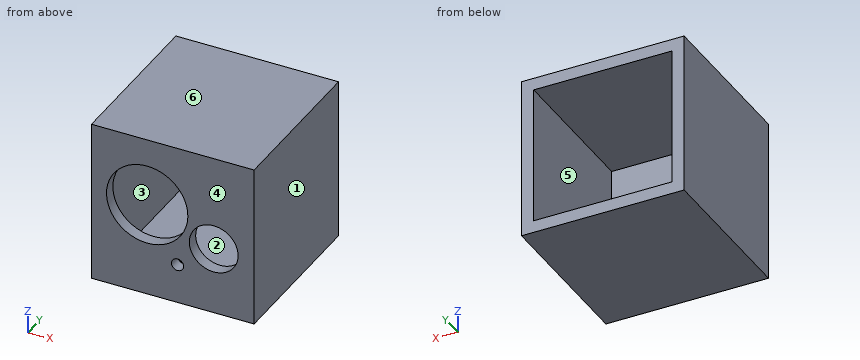
```python
from build123d import *

# Parameters (mm, degrees)
SKETCH1_W           = 20
SKETCH1_H           = 20
BOSS_EXTRUDE1_DEPTH = 20
SHELL1_T            = -1.5
SKETCH2_R           = 5
SKETCH2_R_2         = 0.75
SKETCH2_R_3         = 3
CUT_EXTRUDE1_DEPTH  = 35.641016151


with BuildPart() as part:
    # Sketch1 → Boss-Extrude1 (new body)
    with BuildSketch(Plane(origin=(0, 0, 0), x_dir=(1, 0, 0), z_dir=(0, 1, 0))):
        with Locations((-10, 10)):
            Rectangle(SKETCH1_W, SKETCH1_H)
    extrude(amount=BOSS_EXTRUDE1_DEPTH)

    # Shell1
    shell1_openings = [part.faces().sort_by_distance(p)[0] for p in [
        (-10, 20, -10),
    ]]
    offset(amount=SHELL1_T, openings=shell1_openings, kind=Kind.INTERSECTION)

    # Sketch2 → Cut-Extrude1 (cut, through all)
    with BuildSketch(Plane.XZ):
        with Locations(Location((-13.147042084, -8.401387365, 0), (0, 0, 270))):
            Circle(SKETCH2_R)
        with Locations(Location((-9.417853088, -15.104070699, 0), (0, 0, 270))):
            Circle(SKETCH2_R_2)
        with Locations(Location((-4.966731055, -11.717786539, 0), (0, 0, 270))):
            Circle(SKETCH2_R_3)
    extrude(amount=-CUT_EXTRUDE1_DEPTH, mode=Mode.SUBTRACT)


solid = part.part
```
Source: CAD feature listing. Evaluate the final solid. Frame: model axes, mm. Face numbers are marked on the shaded views. A direction names the side the tool comes from. Coordinates: 2 decimals unless noted, no trailing zeros. Order: outer loops, then holes, each group sorted by start corner. A loop starts at its lowest first (then second) coordinate and runs counter-clockwise, first axis right, second up. Notation, with made-up numbers: M 51,48.25 L 69,48.25 A13 cw 69,73.25 Z; hole C 65,79 d11. An arc over 180 degrees is marked long. Write each question's results on one line, items separated by ' | '. Start each with the question number.
1) Section query D-D (z = -16.5). Return the cut outline in (x, y).
2) Section query B-B (x = -2.75). Return the cut outline in (y, z), plus the area to 3 significant figures.
3) Access query for the marked faces 5 and 6. Directions: +Z, -Z, +X, -X, +Y, -Y. A direction counts if a zero-diameter tool reaches every point of the face in a straight line with its end or side. Return the directions, or none.
4) Section query C-C (z = -5.5). Return the cut outline in (x, y).
5) Line query: line 1 (Z direction, x = -10, y = 16); line 2 (X direction, y = 1, z = -11). Output: solid intervals per line, ascending. Write a range as from..to.
6) Draft query along X for the marked faces 1, 2, 3 and 4. Return one class per face: released by +X, released by -X, zero draft, split by the parting line, or undercut.
7) Section query A-A (y = 6.75). Return the cut outline in (x, z), plus the area to 3 significant figures.
8) Contact query for flat-ended pins moving along their axis: pin 1 Ø5 at (x, y) = (-15.5, 16.5) entering from +Z; pin 2 Ø5 at (x, z) = (-6.5, -11) entering from +Y. Output: stop coordinate, or through.
Answers:
1) outline: M -20,0 L 0,0 L 0,20 L -1.5,20 L -1.5,1.5 L -18.5,1.5 L -18.5,20 L -20,20 Z
2) outline: M 0,-20 L 20,-20 L 20,-18.5 L 1.5,-18.5 L 1.5,-13.74 L 0,-13.74 Z; M 0,-9.7 L 1.5,-9.7 L 1.5,-1.5 L 20,-1.5 L 20,0 L 0,0 Z | area: 79.4 mm^2
3) face 5: +Y | face 6: +Z, +X, -X, +Y, -Y
4) outline: M -20,0 L -17.22,0 L -17.22,1.5 L -18.5,1.5 L -18.5,20 L -20,20 Z; M -9.07,0 L 0,0 L 0,20 L -1.5,20 L -1.5,1.5 L -9.07,1.5 Z
5) line 1: z = -20..-18.5, -1.5..0 | line 2: x = -20..-17.42, -8.88..-7.88, -2.05..0
6) face 1: released by +X | face 2: undercut | face 3: undercut | face 4: zero draft
7) outline: M -20,-20 L 0,-20 L 0,0 L -20,0 Z; hole M -18.5,-18.5 L -1.5,-18.5 L -1.5,-1.5 L -18.5,-1.5 Z | area: 111 mm^2
8) pin 1: stops at z = 0 | pin 2: stops at y = 1.5
